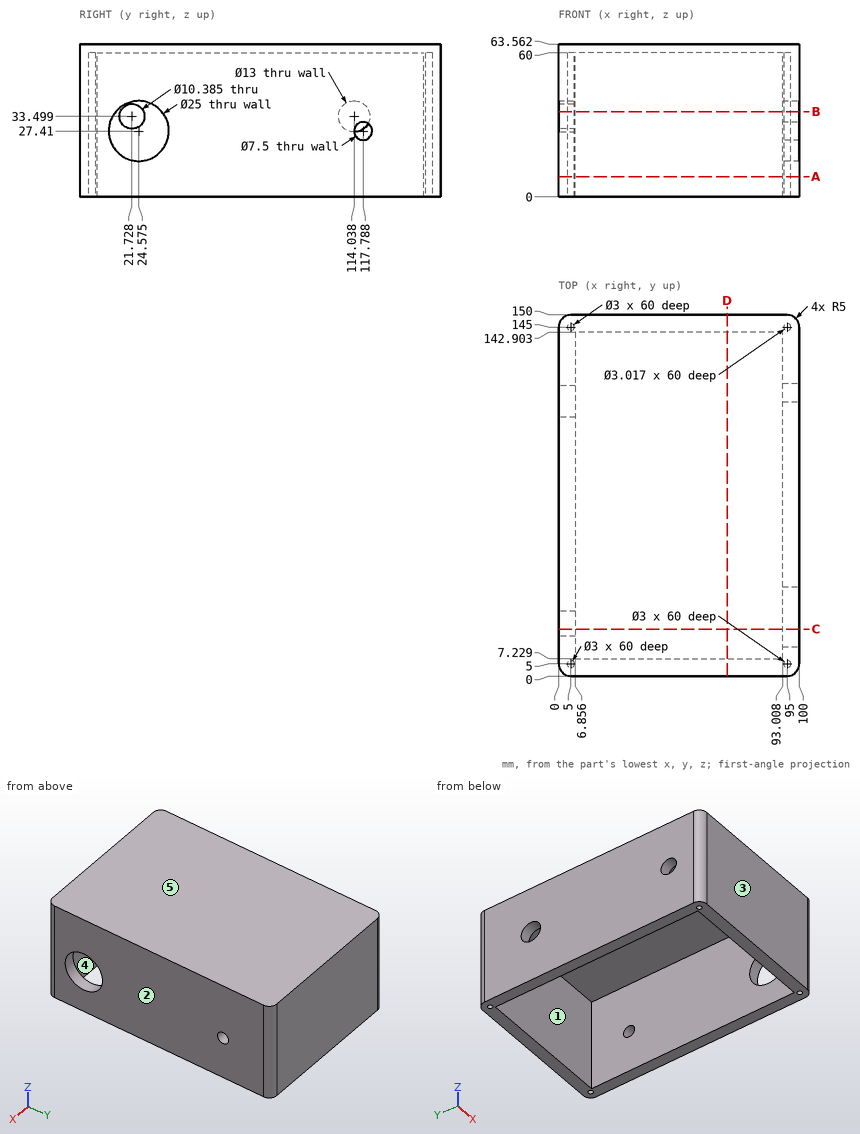
The drawing under review shows one solid part. Ordinate dimensions are in mm from its lowest x, y, z. A direction names the side the tool comes from. Coordinates: 2 decimals unless noted, no trailing zeros. Order: outer loops, then holes, each group sorted by start corner. A loop starts at its lowest first (then second) coordinate and runs counter-clockwise, first axis right, second up. Notation, with made-up numbers: M -21,87 L 6,87 A25 ccw 6,105 Z; hole C -38.5,-24 d7. An arc over 180 degrees is marked long. Use a Markdown table: item, result.
(1) Draft analysis for pull direction X (two halves, no side actions). For the marked faces 1, 2 and 3, state which applies: released by +X, released by -X, zero draft, split by the parting line, or undercut.
Worked answers:
| item | result |
|---|---|
| face 1 | undercut |
| face 2 | released by +X |
| face 3 | zero draft |
(2) For P1, Ø2, axis at x = 42.5, y = 58, coming from the -Z side; P2, Ø5, axis at y = 20, z = 19.5, coming from the +X side; P3, Ø3, axis at y = 112.5, z = 35.5, coming from the -X side, all flat-tipped, find the tip position at first contact; note any pin that passes through.
Worked answers:
| item | result |
|---|---|
| P1 | stops at z = 60 |
| P2 | stops at x = 6.86 |
| P3 | stops at x = 93.01 |
(3) Wall thickness on probe 1 along X at (y, z) = (10, 24.5) (1 decimal); probe 2 along Y at (x, z) = (16.5, 12); probe 3 along X at (y, z) = (145, 35): over which ranges is each line inside the solid? List them lowest first.
Worked answers:
| item | result |
|---|---|
| probe 1 | x = 0 to 6.9, 93 to 100 |
| probe 2 | y = 0 to 7.23, 142.9 to 150 |
| probe 3 | x = 0 to 3.5, 6.5 to 93.49, 96.51 to 100 |
(4) Add section C-C (y = 19.5). Give the boundary of the cut face in (x, z) (1 decimal).
Worked answers:
| item | result |
|---|---|
| outline | M 0,0 L 6.9,0 L 6.9,28.8 L 0,28.8 Z; M 0,38.2 L 6.9,38.2 L 6.9,60 L 93,60 L 93,38.8 L 100,38.8 L 100,63.6 L 0,63.6 Z; M 93,0 L 100,0 L 100,16 L 93,16 Z |
(5) Add section A-A (z = 8.5). Give the boundary of the cut face in (x, y) (1 decimal).
Worked answers:
| item | result |
|---|---|
| outline | M 0,5 A5 ccw 5,0 L 95,0 A5 ccw 100,5 L 100,145 A5 ccw 95,150 L 5,150 A5 ccw 0,145 Z; hole C 5,5 d3; hole C 5,145 d3; hole M 6.9,7.2 L 93,7.2 L 93,142.9 L 6.9,142.9 Z; hole C 95,5 d3; hole C 95,145 d3 |
(6) Add section D-D (x = 70). Give the boundary of the cut face in (y, z), then the cut area to 3 significant figures.
Worked answers:
| item | result |
|---|---|
| outline | M 0,0 L 7.23,0 L 7.23,60 L 142.9,60 L 142.9,0 L 150,0 L 150,63.56 L 0,63.56 Z |
| area | 1,390 mm2 |
(7) Add section B-B (z = 35.5). Give the boundary of the cut face in (x, y) (1 decimal).
Worked answers:
| item | result |
|---|---|
| outline | M 0,5 A5 ccw 5,0 L 95,0 A5 ccw 100,5 L 100,15 L 93,15 L 93,7.2 L 6.9,7.2 L 6.9,16.9 L 0,16.9 Z; M 0,26.5 L 6.9,26.5 L 6.9,107.9 L 0,107.9 Z; M 0,120.2 L 6.9,120.2 L 6.9,142.9 L 93,142.9 L 93,34.1 L 100,34.1 L 100,145 A5 ccw 95,150 L 5,150 A5 ccw 0,145 Z; hole C 5,5 d3; hole C 5,145 d3; hole C 95,5 d3; hole C 95,145 d3 |
(8) For the marked faces 4 and 5, list the 3-axis set-ups (+Z, -Z, +X, -X, +Y, -Y) from which the entire face can be reached by the end or side of a thin tool; tool diameter is ignored.
Worked answers:
| item | result |
|---|---|
| face 4 | -Z |
| face 5 | +Z, +X, -X, +Y, -Y |
